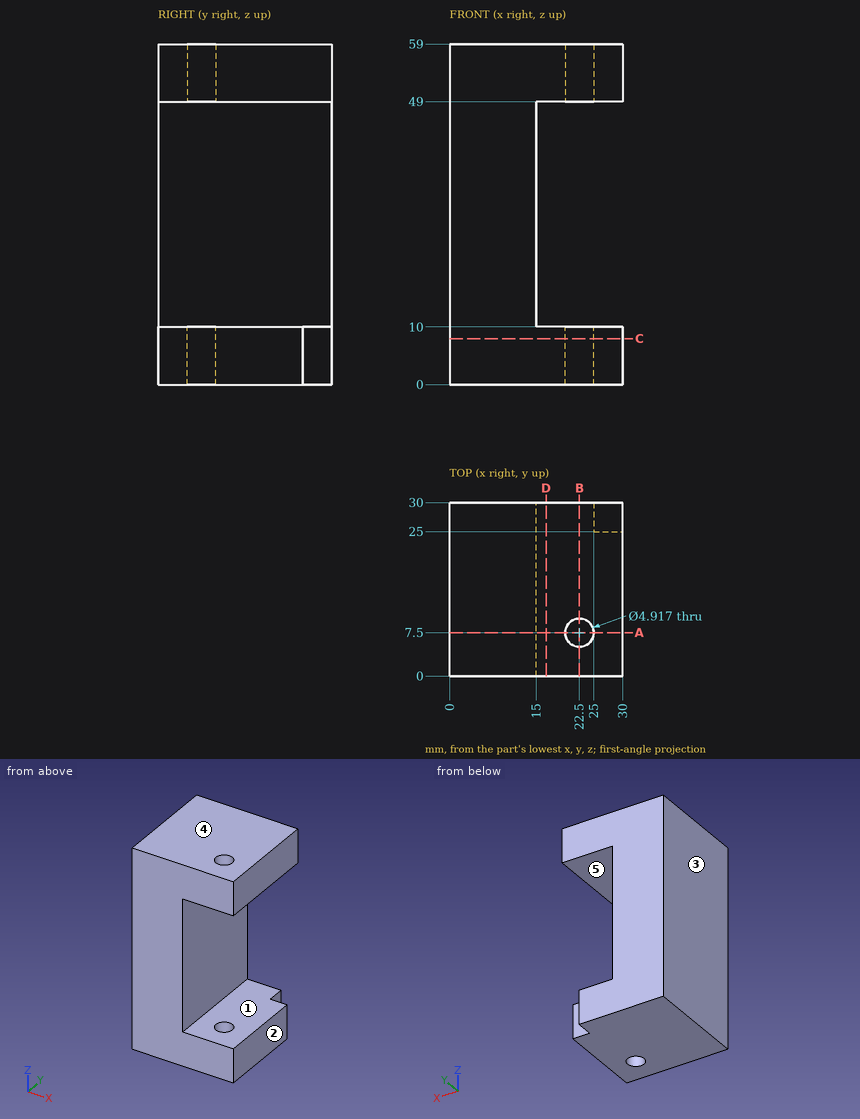
Source: three-view drawing plus pictorial views. Frame: mm from the lowest corner of the part. A direction names the side the tool comes from. Round coordinates to 2 decimals unless told otherwise and drop trailing zeros. Order: outer loops, then holes, each group sorted by start corner. A loop starts at its lowest first (then second) coordinate and runs counter-clockwise, first axis right, second up. Notation, with made-up numbers: (50, 14) - (67, 14) arc R15 ccw to (67, 38) - close; hole circle Ø9 at (31.25, -37.75). An arc over 180 degrees is marked (long way). Use a Markdown table: item, result.
1. First-contact query: pin 1 (1.5 mm diameter, centred on x = 28.5, z = 7, fed in from +Y); pin 2 (4.5 mm diameter, centred on x = 22.5, y = 7.5, fed in from +Z). Flat tips, straight axial feed; report the tip coordinate or a pass-through.
Evaluation:
| item | result |
|---|---|
| pin 1 | y = 25 |
| pin 2 | through |
2. Section C-C on z = 8. Return the cut outline in (x, y), then the cut area to 3 significant figures.
Evaluation:
| item | result |
|---|---|
| outline | (0, 0) - (30, 0) - (30, 25) - (25, 25) - (25, 30) - (0, 30) - close; hole circle Ø4.92 at (22.5, 7.5) |
| area | 856 mm^2 |
3. Section A-A on y = 7.5. Return the cut outline in (x, z).
Evaluation:
| item | result |
|---|---|
| outline | (0, 0) - (20.04, 0) - (20.04, 10) - (15, 10) - (15, 49) - (20.04, 49) - (20.04, 59) - (0, 59) - close; (24.96, 0) - (30, 0) - (30, 10) - (24.96, 10) - close; (24.96, 49) - (30, 49) - (30, 59) - (24.96, 59) - close |
4. Mould query, pull axis Z, two halves, no side actions, for the marked faces 3, 4 and 5. Classes: +Z half, -Z half, draft (parallel to the pull), parting line (faces both ways), or undercut.
Evaluation:
| item | result |
|---|---|
| face 3 | draft |
| face 4 | +Z half |
| face 5 | undercut |
5. Section D-D on x = 16.75. Return the cut outline in (y, z), then the cut area to 3 significant figures.
Evaluation:
| item | result |
|---|---|
| outline | (0, 0) - (30, 0) - (30, 10) - (0, 10) - close; (0, 49) - (30, 49) - (30, 59) - (0, 59) - close |
| area | 600 mm^2 |
6. Access query for the marked faces 1 and 2. Directions: +Z, -Z, +X, -X, +Y, -Y. A direction counts if a zero-diameter tool reaches every point of the face in a straight line with its end or side. Return the directions, or none.
Evaluation:
| item | result |
|---|---|
| face 1 | +X, +Y, -Y |
| face 2 | +Z, -Z, +X, +Y, -Y |
7. Material intervals for probe 1 along Y at (x, z) = (22.5, 3.5); probe 2 along Z at (x, y) = (27.25, 14); probe 3 along X at (y, z) = (7.5, 52), sorted ascending.
Evaluation:
| item | result |
|---|---|
| probe 1 | 0 to 5.04, 9.96 to 30 |
| probe 2 | 0 to 10, 49 to 59 |
| probe 3 | 0 to 20.04, 24.96 to 30 |
8. Section B-B on x = 22.5. Return the cut outline in (y, z).
Evaluation:
| item | result |
|---|---|
| outline | (0, 0) - (5.04, 0) - (5.04, 10) - (0, 10) - close; (0, 49) - (5.04, 49) - (5.04, 59) - (0, 59) - close; (9.96, 0) - (30, 0) - (30, 10) - (9.96, 10) - close; (9.96, 49) - (30, 49) - (30, 59) - (9.96, 59) - close |
